from build123d import *

# Parameters (mm, degrees)
BOSS_EXTRUDE1_DEPTH            = 15
CUT_EXTRUDE1_DEPTH             = 1.5875
CUT_EXTRUDE1_DEPTH_BACK        = 1.5875
CBORE_FOR_M4_SHCS1_D           = 4.5
CBORE_FOR_M4_SHCS1_CBORE_D     = 8
CBORE_FOR_M4_SHCS1_CBORE_DEPTH = 4
CUT_EXTRUDE2_DEPTH             = 26


with BuildPart() as part:
    # Sketch1 → Boss-Extrude1 (new body, symmetric)
    with BuildSketch(Plane(origin=(0, 0, 0), x_dir=(1, 0, 0), z_dir=(0, 1, 0))):
        with BuildLine():
            Line((0, 0), (-15, 0))
            ThreePointArc((-15, 0), (-40, 10.355339059), (-65, 0))
            Line((-65, 0), (-80, 0))
            Line((-80, 0), (-68.342308546, 25))
            Line((-68.342308546, 25), (-14.43375673, 25))
            Line((-14.43375673, 25), (0, 0))
        make_face()
    extrude(amount=BOSS_EXTRUDE1_DEPTH, both=True)

    # Sketch2 → Cut-Extrude1 (cut, two sides)
    with BuildSketch(Plane(origin=(0, 0, 0), x_dir=(1, 0, 0), z_dir=(0, 1, 0))) as cut_extrude1_sk:
        with BuildLine():
            Line((-13.279056191, 3), (-1.732050808, 3))
            Line((-1.732050808, 3), (-14.43375673, 25))
            Line((-14.43375673, 25), (-68.342308546, 25))
            Line((-68.342308546, 25), (-73.005385128, 15))
            Line((-73.005385128, 15), (-22.040346526, 15))
            ThreePointArc((-22.040346526, 15), (-20.452846526, 14.574630657), (-19.290715869, 13.4125))
            Line((-19.290715869, 13.4125), (-13.279056191, 3))
        make_face()
    extrude(amount=CUT_EXTRUDE1_DEPTH, mode=Mode.SUBTRACT)
    extrude(cut_extrude1_sk.sketch, amount=-CUT_EXTRUDE1_DEPTH_BACK, mode=Mode.SUBTRACT)

    # CBORE for M4 SHCS1 (through all)
    with Locations(Plane(origin=(0, 15, 0), x_dir=(1, 0, 0), z_dir=(0, 1, 0))):
        with Locations((-59.43375673, 20), (-19.43375673, 20)):
            CounterBoreHole(CBORE_FOR_M4_SHCS1_D / 2, CBORE_FOR_M4_SHCS1_CBORE_D / 2, CBORE_FOR_M4_SHCS1_CBORE_DEPTH)

    # Sketch7 → Cut-Extrude2 (cut, through all)
    with BuildSketch(Plane.XY):
        Polygon((0, 5), (-15, 15), (0, 15), align=None)
        Polygon((0, -15), (-15, -15), (0, -5), align=None)
    extrude(amount=-CUT_EXTRUDE2_DEPTH, mode=Mode.SUBTRACT)


solid = part.part
Input: part model. Units: mm. Frame: model coordinates. A direction names the side the tool comes from. Round coordinates to 2 decimals unless told otherwise and drop trailing zeros. Loops run counter-clockwise (first coordinate to the right, second up) from the corner with the lowest first, then second, coordinate; pieces in that order, holes last. Notation, with made-up numbers: (-36, 7.25) -> (14, 7.25) arc R17 ccw to (14, 22.25) -> close; hole circle Ø8 at (-17.5, 67). An arc over 180 degrees is marked (long way). Answer as a JSON object with one key per item and string values. Group by question number.
1) Section query D-D on z = -20. State how many separate pieces and enclosed holes the cut face has, plus the area to 3 significant figures.
2) Pin query (flat end, axial travel): pin 1 (2 mm diameter, centred on y = 3.5, z = -19.5, fed in from +X); pin 2 (7 mm diameter, centred on x = -19.43, z = -20, fed in from +Y); pin 3 (5 mm diameter, centred on y = -11, z = -11, fed in from -X). Return the tip coordinate at first contact, or that it passes through.
3) Section query C-C on x = -27. Output: boundary loops of the cut face in (y, z), plus the area to 3 significant figures.
4) Ray query, L1, parallel to X at y = -10, z = -20; L2, parallel to Y at x = -24, z = -19.5; L3, parallel to X at y = -7.5, z = -2.75. Return the intervals inside material, ascending.
5) Section query A-A on z = -9.25. Output: boundary loops of the cut face in (x, y).
6) Draft query along Y for faces 1 (the flat face through (-42, 8, -25)), 2 (the cylindrical face through (-20.5, 0, -14.6)), 3 (the flat face through (-18, 11, -18)). Return one class per face: +Y half, -Y half, draft (parallel to the pull), parting line (faces both ways), or undercut.
7) Reachability of faces 4 (the flat face through (-38, -1.588, -19)), 5 (the flat face through (-58, 11, -18)), 6 (the flat face through (-48, 0, -15)), 7 (the flat face through (-74.253, 0.21, -12.325)), 8 (the flat face through (-9, 11, -10)) from +Z, -Z, +X, -X, +Y, -Y: full face, straight path, thin tool, end or side. Return the list, or none.
8) Section query B-B on y = -10.5. Output: boundary loops of the cut face in (x, z), plus the area to 3 significant figures.
Reply:
{
 "1": {"separate pieces": "6", "enclosed holes": "0", "area": "1,310 mm2"},
 "2": {"pin 1": "stops at x = -10.68", "pin 2": "stops at y = 11", "pin 3": "stops at x = -76.04"},
 "3": {"outline": "(-15, -25) -> (-1.59, -25) -> (-1.59, -15) -> (1.59, -15) -> (1.59, -25) -> (15, -25) -> (15, -7.88) -> (-15, -7.88) -> close", "area": "482 mm2"},
 "4": {"L1": "x = -70.67 to -61.68, -57.18 to -21.68, -17.18 to -11.55", "L2": "y = -15 to -1.59, 1.59 to 15", "L3": "x = -78.72 to -61.91, -18.09 to -3.75"},
 "5": {"outline": "(-75.69, -15) -> (-48.77, -15) -> (-48.77, 15) -> (-75.69, 15) -> close; (-31.23, -15) -> (-15, -15) -> (-5.34, -8.56) -> (-5.34, -1.59) -> (-16.89, -1.59) -> (-16.89, 1.59) -> (-5.34, 1.59) -> (-5.34, 8.56) -> (-15, 15) -> (-31.23, 15) -> close"},
 "6": {"face 1": "draft", "face 2": "undercut", "face 3": "+Y half"},
 "7": {"face 4": "-Z, +X", "face 5": "+Y", "face 6": "-Z, +X, -X", "face 7": "-Z, -X, +Y, -Y", "face 8": "+Z, -Z, +X, +Y"},
 "8": {"outline": "(-80, 0) -> (-68.34, -25) -> (-14.43, -25) -> (-8.25, -14.29) -> (-8.25, 0) -> (-15, 0) arc R35.36 cw to (-65, 0) -> close; hole circle Ø4.5 at (-59.43, -20); hole circle Ø4.5 at (-19.43, -20)", "area": "1,230 mm2"}
}
